Read the model definition and answer for the solid it produces. Units are mm, in the model's axes. Face numbers are marked on the shaded views. A direction names the side the tool comes from. Give positions to 0.01 mm unless a question says otherwise; leave off trailing zeros. Loops run counter-clockwise (first coordinate to the right, second up) from the corner with the lowest first, then second, coordinate; pieces in that order, holes last.
(1) Determine the mould class of the marked faces 1, 2 and 3 for opening direction Y: pulls with the +Y half, pulls with the -Y half, needs draft (parallel to the pull), parting line crosses it, or undercut.
(2) Straight lines are drawn through the part: probe 1 along Y at (x, z) = (-3.7, -19.05); probe 2 along Y at (x, z) = (9, -17); probe 3 along X at (y, z) = (165.1, 3.1) (1 decimal). For each, find the intervals that lie inside material, in ascending order.
(3) Each of these flat-tipped pins is pushed along its axis until it touches: P1, Ø12.5, axis at x = 7.94, y = 165.1, coming from the -Z side; P2, Ø5, axis at x = 12, y = 133.5, coming from the -Z side; P3, Ø12, axis at x = 9, z = -1.5, coming from the -Y side; P4, Ø1, axis at x = 3, z = -5, coming from the -Y side. Where does it stop, or does it pass through?
(4) Find section D-D, the plane z = -2.5. Write down the section's boundary in (x, y), then the cut area to 3 significant figures.
(5) Which of the six approach directions +Z, -Z, +X, -X, +Y, -Y give full straight-line access (tool end or side, diameter ignored) to the marked faces 4, 5, 6, 7 and 8?
(6) Find section B-B, the plane y = 101.6. Write down the section's boundary in (x, z), then the cut area to 3 significant figures.
(7) Find section A-A, the plane z = -19.05. Write down the section's boundary in (x, y).
```python
from build123d import *

# Parameters (mm, degrees)
SKETCH2_W           = 31.75
SKETCH2_H           = 152.4
SKETCH2_R           = 4.7625
BOSS_EXTRUDE1_DEPTH = 4.7625
SKETCH3_W           = 26.07038402
SKETCH3_H           = 203.2
SKETCH3_R           = 4.7625
BOSS_EXTRUDE2_DEPTH = 4.7625
SKETCH4_W           = 21.30788402
SKETCH4_H           = 25.4
BOSS_EXTRUDE3_DEPTH = 25.4


with BuildPart() as part:
    # Sketch2 → Boss-Extrude1 (new body)
    with BuildSketch(Plane(origin=(0, 0, 0), x_dir=(0, 0, -1), z_dir=(1, 0, 0))):
        with Locations((15.875, 76.2)):
            Rectangle(SKETCH2_W, SKETCH2_H)
        with Locations((19.05, 101.6)):
            Circle(SKETCH2_R, mode=Mode.SUBTRACT)
    extrude(amount=-BOSS_EXTRUDE1_DEPTH)

    # Sketch3 → Boss-Extrude2 (add)
    with BuildSketch(Plane.XY):
        with Locations((8.27269201, 76.2)):
            Rectangle(SKETCH3_W, SKETCH3_H)
        with Locations(Location((7.9375, 165.1, 0), (0, 0, 180))):
            Circle(SKETCH3_R, mode=Mode.SUBTRACT)
        with Locations(Location((8.60788402, -12.7, 0), (0, 0, 180))):
            Circle(SKETCH3_R, mode=Mode.SUBTRACT)
    extrude(amount=BOSS_EXTRUDE2_DEPTH)

    # Sketch4 → Boss-Extrude3 (add)
    with BuildSketch(Plane(origin=(0, 0, 0), x_dir=(-1, 0, 0), z_dir=(0, 0, -1))):
        with Locations((-10.65394201, 139.7)):
            Rectangle(SKETCH4_W, SKETCH4_H)
        with Locations((-10.65394201, 12.7)):
            Rectangle(SKETCH4_W, SKETCH4_H)
    extrude(amount=BOSS_EXTRUDE3_DEPTH)


solid = part.part
```
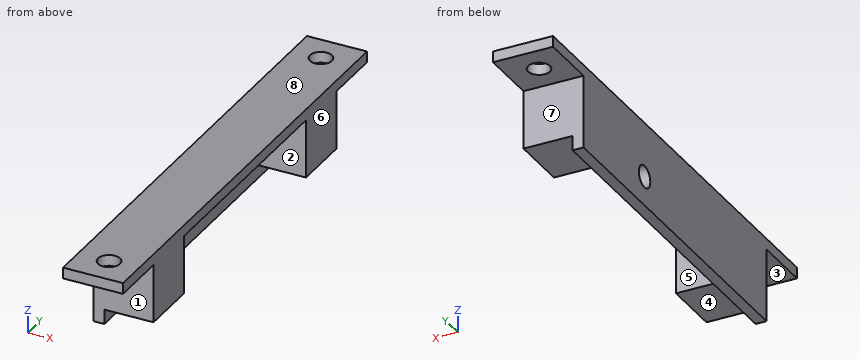
Entries:
1. face 1: pulls with the -Y half
1. face 2: undercut
1. face 3: needs draft
2. probe 1: y = 0 to 96.84, 106.36 to 152.4
2. probe 2: y = 0 to 25.4, 127 to 152.4
2. probe 3: x = -4.8 to 3.2, 12.7 to 21.3
3. P1: stops at z = 0
3. P2: stops at z = -25.4
3. P3: stops at y = -25.4
3. P4: stops at y = 0
4. outline: (-4.76, 0) - (21.31, 0) - (21.31, 25.4) - (0, 25.4) - (0, 127) - (21.31, 127) - (21.31, 152.4) - (-4.76, 152.4) - close
4. area: 1,810 mm2
5. face 4: -Z, +X, +Y, -Y
5. face 5: -Z, +X
5. face 6: +Z, -Z, +X, +Y, -Y
5. face 7: -Z, +X, -X, +Y
5. face 8: +Z, +X, -X, +Y, -Y
6. outline: (-4.76, -31.75) - (0, -31.75) - (0, -23.81) - (-4.76, -23.81) - close; (-4.76, -14.29) - (0, -14.29) - (0, 0) - (21.31, 0) - (21.31, 4.76) - (-4.76, 4.76) - close
6. area: 230 mm2
7. outline: (-4.76, 0) - (21.31, 0) - (21.31, 25.4) - (0, 25.4) - (0, 96.84) - (-4.76, 96.84) - close; (-4.76, 106.36) - (0, 106.36) - (0, 127) - (21.31, 127) - (21.31, 152.4) - (-4.76, 152.4) - close
